Build history of the part. All positions in model axes, mm. A direction names the side the tool comes from. Give positions to 0.01 mm unless a question says otherwise; leave off trailing zeros. Order: outer loops, then holes, each group sorted by start corner. A loop starts at its lowest first (then second) coordinate and runs counter-clockwise, first axis right, second up. Notation, with made-up numbers: M -8,78.5 L 9,78.5 A19 ccw 9,94.5 Z; hole C 38,69 d1. An arc over 180 degrees is marked long. One line per item, written item: value.
from build123d import *

# Parameters (mm, degrees)
EXTRUDE_1_DEPTH     = 40
SKETCH_3_R          = 2.5
CUT_EXTRUDE_1_DEPTH = 44.127717306
SKETCH_5_OUTSIDE_W  = 39.896
SKETCH_5_OUTSIDE_H  = 51.896
CUT_EXTRUDE_3_DEPTH = 44.127717449
CUT_EXTRUDE_4_DEPTH = 4
MOVE_BODY_1_ANGLE   = 48
SKETCH_7_OUTSIDE_W  = 45.818
SKETCH_7_OUTSIDE_H  = 48.186
CUT_EXTRUDE_6_DEPTH = 50


with BuildPart() as part:
    # 草图2 → 凸台-拉伸1 (new body)
    with BuildSketch(Plane.XY):
        with BuildLine():
            Line((14, 0), (-14, 0))
            Line((-14, 0), (-14, 4))
            ThreePointArc((-14, 4), (-12.828427125, 6.828427125), (-10, 8))
            Line((-10, 8), (10, 8))
            ThreePointArc((10, 8), (12.828427125, 6.828427125), (14, 4))
            Line((14, 4), (14, 0))
        make_face()
    extrude(amount=-EXTRUDE_1_DEPTH)

    # 草图3 → 切除-拉伸1 (cut, through all)
    with BuildSketch(Plane(origin=(0, 0, 0), x_dir=(1, 0, 0), z_dir=(0, 1, 0))):
        with Locations(Location((-9, 35, 0), (0, 0, 113.578178478))):
            Circle(SKETCH_3_R)
        with Locations(Location((9, 35, 0), (0, 0, 66.421821522))):
            Circle(SKETCH_3_R)
        with Locations(Location((-9, 5, 0), (0, 0, 113.578178478))):
            Circle(SKETCH_3_R)
        with Locations(Location((9, 5, 0), (0, 0, 66.421821522))):
            Circle(SKETCH_3_R)
    extrude(amount=CUT_EXTRUDE_1_DEPTH, mode=Mode.SUBTRACT)

    # 草图5 outside → 切除-拉伸3 (cut, through all)
    with BuildSketch(Plane(origin=(0, 8, 0), x_dir=(1, 0, 0), z_dir=(0, 1, 0))):
        with Locations((0, 20)):
            Rectangle(SKETCH_5_OUTSIDE_W, SKETCH_5_OUTSIDE_H)
        with BuildLine():
            Line((14, 5), (14, 35))
            ThreePointArc((14, 35), (12.535533906, 38.535533906), (9, 40))
            Line((9, 40), (-9, 40))
            ThreePointArc((-9, 40), (-12.535533906, 38.535533906), (-14, 35))
            Line((-14, 35), (-14, 5))
            ThreePointArc((-14, 5), (-12.535533906, 1.464466094), (-9, 0))
            Line((-9, 0), (9, 0))
            ThreePointArc((9, 0), (12.535533906, 1.464466094), (14, 5))
        make_face(mode=Mode.SUBTRACT)
    extrude(amount=-CUT_EXTRUDE_3_DEPTH, mode=Mode.SUBTRACT)

    # 草图6 → 切除-拉伸4 (cut)
    with BuildSketch(Plane.XZ):
        with BuildLine():
            Line((14, -26), (-2, -26))
            ThreePointArc((-2, -26), (-8, -20), (-2, -14))
            Line((-2, -14), (14, -14))
            ThreePointArc((14, -14), (20, -20), (14, -26))
        make_face()
    extrude(amount=-CUT_EXTRUDE_4_DEPTH, mode=Mode.SUBTRACT)


with BuildPart() as part_1:
    # Move Body 1: moved
    add(part.part.rotate(Axis((0, 4, -20), (-1, 0, 0)), MOVE_BODY_1_ANGLE))

    # 草图7 outside → 切除-拉伸6 (cut)
    with BuildSketch(Plane.ZY.offset(14)):
        with Locations((-20, 4)):
            Rectangle(SKETCH_7_OUTSIDE_W, SKETCH_7_OUTSIDE_H)
        with BuildLine():
            Line((-6.990461603, 12.470649957), (-3.644808571, 16.186374084))
            Line((-3.644808571, 16.186374084), (-8.103677524, 20.201157722))
            ThreePointArc((-8.103677524, 20.201157722), (-9.546610649, 20.712127141), (-10.928228387, 20.053129284))
            Line((-10.928228387, 20.053129284), (-11.40244938, 19.526453515))
            Line((-11.40244938, 19.526453515), (-14.468791033, 16.1209361))
            Line((-14.468791033, 16.1209361), (-31.476367571, -2.767891249))
            Line((-31.476367571, -2.767891249), (-34.542709224, -6.173408664))
            Line((-34.542709224, -6.173408664), (-35.016930216, -6.700084433))
            ThreePointArc((-35.016930216, -6.700084433), (-35.527899635, -8.143017558), (-34.868901778, -9.524635297))
            Line((-34.868901778, -9.524635297), (-30.410032825, -13.539418935))
            Line((-30.410032825, -13.539418935), (-27.064379793, -9.823694808))
            Line((-27.064379793, -9.823694808), (-6.990461603, 12.470649957))
        make_face(mode=Mode.SUBTRACT)
    extrude(amount=-CUT_EXTRUDE_6_DEPTH, mode=Mode.SUBTRACT)


solid = part_1.part
1) Mould opens along Z. For faces 4 (the face through (-8, 3, -19)), 5 (the face through (-0.164, 20.713, -9.525)), 6 (the face through (14, 11, -11)) say: released by +Z, released by -Z, zero draft, split by the parting line, or undercut.
Check values:
face 4: undercut
face 5: split by the parting line
face 6: zero draft
2) Saw through at B-B, the plane z = -29.5. Give the number of separate pieces and of enclosed holes in the cut face, then the cut area to 3 significant figures.
Check values:
separate pieces: 1
enclosed holes: 2
area: 267 mm^2
3) Saw through at A-A, the plane x = -5.25. Write the cut outline in (y, z).
Check values:
outline: M -13.54,-30.41 L -9.52,-34.87 A2 ccw -6.7,-35.02 L 20.05,-10.93 A2 ccw 20.2,-8.1 L 16.19,-3.64 L 5.07,-13.65 L 7.75,-16.63 L 0.25,-23.37 L -2.42,-20.4 Z
4) Drill centre lines: probe 1 along X at (y, z) = (16.5, -12.5); probe 2 along Y at (x, z) = (-3.5, -23); probe 3 along Z at (x, y) = (-7.5, -8). Where is each one in solid material? Low to high. Write a range as from..to.
Check values:
probe 1: -12.87..-11.4, -6.6..6.6, 11.4..12.87
probe 2: -5.31..-1.12, 0.67..6.65
probe 3: -35.53..-32.08, -26.1..-25.42
5) Tool access for faces 1 (the face through (5.888, 7.102, -14.478)), 2 (the face through (6.112, -1.816, -22.508)), 3 (the face through (-14, 3, -18)): list every direction of +Z, -Z, +X, -X, +Y, -Y with a clear straight run to the whole face (end or side of a thin tool).
Check values:
face 1: +X, -Y
face 2: +Z, +X
face 3: +Z, -Z, -X, +Y, -Y
6) Pin check, flat tips, straight feed: pin 1 (8 mm diameter, centred on x = 3, z = -8.5, fed in from -Y); pin 2 (6 mm diameter, centred on x = -1.5, z = -20.5, fed in from -Y); pin 3 (10 mm diameter, centred on y = 15.5, z = -20.5, fed in from -X). Stop position of each tip, or through.
Check values:
pin 1: y = 6.35
pin 2: y = -5.87
pin 3: x = -12.57
